For this review, take the finished solid that the model builds, in its own axes (mm). Round coordinates to 2 decimals unless told otherwise and drop trailing zeros. Loops run counter-clockwise (first coordinate to the right, second up) from the corner with the lowest first, then second, coordinate; pieces in that order, holes last.
1. Consider section A-A on z = 12.7. State the section outline as (x, y) points, then the cut area to 3 significant figures.
2. Consider section C-C on y = 16.25. State the section outline as (x, z) points.
3. Consider section B-B on x = 30.5. State the section outline as (y, z) points.
4. To check wall thickness, follow line 1 along Y through (x, z) = (24, 12.55); line 2 along X through (y, z) = (10.5, 14); line 3 along Y through (x, z) = (8, 13.5). State the ranges of each line that lie inside material, in increasing order.
5. Draft analysis for pull direction Y (two halves, no side actions). For faces 1 (the cylindrical face through (8.48, 23.93, 11.6)), 2 (the flat face through (7, 17, 13)), 3 (the cylindrical face through (8.52, 26.25, 14.36)), state which applies: released by +Y, released by -Y, zero draft, split by the parting line, or undercut.
6. Clearance check with flat-ended pins moving along their axes: pin 1 Ø1.5 at (x, z) = (21, 11.5) entering from +Y; pin 2 Ø1.5 at (x, z) = (36.5, 11.5) entering from -Y; pin 3 Ø1.2 at (y, z) = (13, 12.5) entering from -X. State where each tip first meets the part, or that it passes through.
from build123d import *
from build123d.topology import SkipClean

# Parameters (mm, degrees)
SKETCH1_R           = 2
BOSS_EXTRUDE1_DEPTH = 42
BOSS_EXTRUDE2_DEPTH = 10
CUT_EXTRUDE1_DEPTH  = 7
BOSS_EXTRUDE4_DEPTH = 3
SKETCH5_R           = 1.5
CUT_EXTRUDE3_DEPTH  = 54.708670792
SKETCH6_W           = 11.822480184
SKETCH6_H           = 12.15707868
CUT_EXTRUDE5_DEPTH  = 54.708670792
FILLET4_R           = 1
FILLET5_R           = 1


with BuildPart() as part:
    # Sketch1 → Boss-Extrude1 (new body)
    with BuildSketch(Plane(origin=(0, 0, 0), x_dir=(0, 0, -1), z_dir=(1, 0, 0))):
        with Locations(Location((-12.6584653, 7.000514901, 0), (0, 0, 180))):
            Circle(SKETCH1_R)
    extrude(amount=BOSS_EXTRUDE1_DEPTH)

    # Sketch2 → Boss-Extrude2 (add)
    with BuildSketch(Plane.ZY):
        with BuildLine():
            Line((10.6584653, 7.000514901), (10.6584653, 13.760469307))
            ThreePointArc((10.6584653, 13.760469307), (12.6584653, 15.760469307), (14.6584653, 13.760469307))
            Line((14.6584653, 13.760469307), (14.6584653, 7.000514901))
            ThreePointArc((14.6584653, 7.000514901), (12.6584653, 5.000514901), (10.6584653, 7.000514901))
        make_face()
    extrude(amount=-BOSS_EXTRUDE2_DEPTH)

    # Sketch3 → Cut-Extrude1 (cut)
    with SkipClean():  # the faces are left unmerged after this step: merging them gives an invalid solid
        with BuildSketch(Plane.ZY):
            with BuildLine():
                Line((10.6584653, 7.000514901), (10.6584653, 13.760469307))
                ThreePointArc((10.6584653, 13.760469307), (12.6584653, 15.760469307), (14.6584653, 13.760469307))
                Line((14.6584653, 13.760469307), (14.6584653, 7.000514901))
                ThreePointArc((14.6584653, 7.000514901), (12.6584653, 9.000514901), (10.6584653, 7.000514901))
            make_face()
        extrude(amount=-CUT_EXTRUDE1_DEPTH, mode=Mode.SUBTRACT)

    # Sketch4 → Boss-Extrude4 (add)
    with SkipClean():  # the faces are left unmerged after this step: merging them gives an invalid solid
        with BuildSketch(Plane.ZY.offset(-7)):
            with BuildLine():
                Line((10.6584653, 36.009876522), (10.6584653, 13.760469307))
                ThreePointArc((10.6584653, 13.760469307), (12.6584653, 15.760469307), (14.6584653, 13.760469307))
                Line((14.6584653, 13.760469307), (14.6584653, 36.009876522))
                Line((14.6584653, 36.009876522), (10.6584653, 36.009876522))
            make_face()
            with BuildLine():
                ThreePointArc((10.6584653, 36.009876522), (12.6584653, 38.009876522), (14.6584653, 36.009876522))
                Line((14.6584653, 36.009876522), (10.6584653, 36.009876522))
            make_face()
        extrude(amount=-BOSS_EXTRUDE4_DEPTH)

    # Sketch5 → Cut-Extrude3 (cut, through all)
    with SkipClean():  # the faces are left unmerged after this step: merging them gives an invalid solid
        with BuildSketch(Plane.ZY.offset(-7)):
            with Locations((12.706639089, 22.91954594)):
                Circle(SKETCH5_R)
        extrude(amount=-CUT_EXTRUDE3_DEPTH, mode=Mode.SUBTRACT)

    # Sketch6 → Cut-Extrude5 (cut, through all)
    with SkipClean():  # the faces are left unmerged after this step: merging them gives an invalid solid
        with BuildSketch(Plane.ZY.offset(-7)):
            with Locations((12.630555797, 32.616849438)):
                Rectangle(SKETCH6_W, SKETCH6_H)
        extrude(amount=-CUT_EXTRUDE5_DEPTH, mode=Mode.SUBTRACT)

    # Fillet4
    fillet4_edges = [part.edges().sort_by_distance(p)[0] for p in [
        (8.5, 26.538310098, 14.6584653),
    ]]
    fillet(fillet4_edges, radius=FILLET4_R)

    # Fillet5
    fillet5_edges = [part.edges().sort_by_distance(p)[0] for p in [
        (8.5, 26.538310098, 10.6584653),
    ]]
    fillet(fillet5_edges, radius=FILLET5_R)


solid = part.part
Resolved:
1. outline: (0, 5) - (42, 5) - (42, 9) - (10, 9) - (10, 21.42) - (7, 21.42) - (7, 9) - (0, 9) - close; (7, 24.42) - (10, 24.42) - (10, 26.54) - (7, 26.54) - close
1. area: 212 mm2
2. outline: (7, 10.66) - (10, 10.66) - (10, 14.66) - (7, 14.66) - close
3. outline: circle Ø4 at (7, 12.66)
4. line 1: y = 5 to 9
4. line 2: x = 7 to 10
4. line 3: y = 5.19 to 21.65, 24.19 to 26.54
5. face 1: undercut
5. face 2: zero draft
5. face 3: released by +Y
6. pin 1: stops at y = 8.96
6. pin 2: stops at y = 5.04
6. pin 3: stops at x = 7
